Model file for the job. Use its own axes, mm. Round coordinates to 2 decimals unless told otherwise and drop trailing zeros. Loops run counter-clockwise (first coordinate to the right, second up) from the corner with the lowest first, then second, coordinate; pieces in that order, holes last. Notation, with made-up numbers: (-17, 41) - (42, 41) arc R21 ccw to (42, 52) - close; hole circle Ø2 at (23, 59.5). An arc over 180 degrees is marked (long way). Use one line per item in the form item = value.
from build123d import *

# Parameters (mm, degrees)
F1_DEPTH      = 19.05
F2_R          = 3.175
F3_DEPTH      = 19.05
F4_R          = 3.175
F4_R_2        = 1.175
F5_DEPTH      = 304.8
F5_DEPTH_BACK = 19.05


with BuildPart() as f1:
    # F0 (on Top) → F1 (new body)
    with BuildSketch(Plane.XY):
        Polygon((134.8747963854, 77.87), (0, 155.74), (-134.8747963854, 77.87), (-134.8747963854, -77.87), (0, -155.74), (134.8747963854, -77.87), align=None)
    extrude(amount=F1_DEPTH)

    # F2 (on face) → F3 (cut)
    with BuildSketch(Plane.XY.offset(19.05)):
        with BuildLine():
            ThreePointArc((25.4095597529, 94.8297679959), (21.5209947863, 92.5847039657), (23.7660588165, 88.696138999))
            Line((23.7660588165, 88.696138999), (24.5878092847, 91.7629534975))
            Line((24.5878092847, 91.7629534975), (25.4095597529, 94.8297679959))
        make_face()
        with BuildLine():
            ThreePointArc((35.5273806378, 120.7407282861), (30.4195631007, 123.2596251416), (31.5306301696, 117.6739137877))
            ThreePointArc((31.5306301696, 117.6739137877), (34.2851981749, 118.2218314307), (35.5273806378, 120.7407282861))
        make_face()
        with BuildLine():
            Line((24.5878092847, 91.7629534975), (23.7660588165, 88.696138999))
            ThreePointArc((23.7660588165, 88.696138999), (26.5206268218, 89.244056642), (27.7628092847, 91.7629534975))
            ThreePointArc((27.7628092847, 91.7629534975), (27.1067061402, 93.6957710346), (25.4095597529, 94.8297679959))
            Line((25.4095597529, 94.8297679959), (24.5878092847, 91.7629534975))
        make_face()
        with Locations((-24.5878092847, 91.7629534975)):
            Circle(F2_R)
        with Locations((-32.3523806378, 120.7407282861)):
            Circle(F2_R)
        with Locations((-67.1751442127, 67.1751442127)):
            Circle(F2_R)
        with Locations((-88.3883476483, 88.3883476483)):
            Circle(F2_R)
        with Locations((-91.7629534975, 24.5878092847)):
            Circle(F2_R)
        with Locations((-120.7407282861, 32.3523806378)):
            Circle(F2_R)
        with Locations((-91.7629534975, -24.5878092847)):
            Circle(F2_R)
        with Locations((-120.7407282861, -32.3523806378)):
            Circle(F2_R)
        with Locations((-67.1751442127, -67.1751442127)):
            Circle(F2_R)
        with Locations((-88.3883476483, -88.3883476483)):
            Circle(F2_R)
        with Locations((-24.5878092847, -91.7629534975)):
            Circle(F2_R)
        with Locations((-32.3523806378, -120.7407282861)):
            Circle(F2_R)
        with Locations((24.5878092847, -91.7629534975)):
            Circle(F2_R)
        with Locations((32.3523806378, -120.7407282861)):
            Circle(F2_R)
        with Locations((67.1751442127, -67.1751442127)):
            Circle(F2_R)
        with Locations((88.3883476483, -88.3883476483)):
            Circle(F2_R)
        with Locations((91.7629534975, -24.5878092847)):
            Circle(F2_R)
        with Locations((120.7407282861, -32.3523806378)):
            Circle(F2_R)
        with Locations((91.7629534975, 24.5878092847)):
            Circle(F2_R)
        with Locations((120.7407282861, 32.3523806378)):
            Circle(F2_R)
        with Locations((67.1751442127, 67.1751442127)):
            Circle(F2_R)
        with Locations((88.3883476483, 88.3883476483)):
            Circle(F2_R)
    extrude(amount=-F3_DEPTH, mode=Mode.SUBTRACT)

    # F4 (on face) → F5 (join, two sides)
    with BuildSketch(Plane.XY.offset(19.05)) as f5_sk:
        with Locations((-88.3883476483, 88.3883476483)):
            Circle(F4_R)
        with Locations((-88.3883476483, 88.3883476483)):
            Circle(F4_R_2, mode=Mode.SUBTRACT)
        with Locations((-67.1751442127, 67.1751442127)):
            Circle(F4_R)
        with Locations((-67.1751442127, 67.1751442127)):
            Circle(F4_R_2, mode=Mode.SUBTRACT)
        with Locations((-120.7407282861, 32.3523806378)):
            Circle(F4_R)
        with Locations((-120.7407282861, 32.3523806378)):
            Circle(F4_R_2, mode=Mode.SUBTRACT)
        with Locations((-91.7629534975, 24.5878092847)):
            Circle(F4_R)
        with Locations((-91.7629534975, 24.5878092847)):
            Circle(F4_R_2, mode=Mode.SUBTRACT)
        with Locations((-120.7407282861, -32.3523806378)):
            Circle(F4_R)
        with Locations((-120.7407282861, -32.3523806378)):
            Circle(F4_R_2, mode=Mode.SUBTRACT)
        with Locations((-91.7629534975, -24.5878092847)):
            Circle(F4_R)
        with Locations((-91.7629534975, -24.5878092847)):
            Circle(F4_R_2, mode=Mode.SUBTRACT)
        with Locations((-88.3883476483, -88.3883476483)):
            Circle(F4_R)
        with Locations((-88.3883476483, -88.3883476483)):
            Circle(F4_R_2, mode=Mode.SUBTRACT)
        with Locations((-67.1751442127, -67.1751442127)):
            Circle(F4_R)
        with Locations((-67.1751442127, -67.1751442127)):
            Circle(F4_R_2, mode=Mode.SUBTRACT)
        with Locations((-32.3523806378, -120.7407282861)):
            Circle(F4_R)
        with Locations((-32.3523806378, -120.7407282861)):
            Circle(F4_R_2, mode=Mode.SUBTRACT)
        with Locations((-24.5878092847, -91.7629534975)):
            Circle(F4_R)
        with Locations((-24.5878092847, -91.7629534975)):
            Circle(F4_R_2, mode=Mode.SUBTRACT)
        with Locations((32.3523806378, -120.7407282861)):
            Circle(F4_R)
        with Locations((32.3523806378, -120.7407282861)):
            Circle(F4_R_2, mode=Mode.SUBTRACT)
        with Locations((24.5878092847, -91.7629534975)):
            Circle(F4_R)
        with Locations((24.5878092847, -91.7629534975)):
            Circle(F4_R_2, mode=Mode.SUBTRACT)
        with Locations((88.3883476483, -88.3883476483)):
            Circle(F4_R)
        with Locations((88.3883476483, -88.3883476483)):
            Circle(F4_R_2, mode=Mode.SUBTRACT)
        with Locations((67.1751442127, -67.1751442127)):
            Circle(F4_R)
        with Locations((67.1751442127, -67.1751442127)):
            Circle(F4_R_2, mode=Mode.SUBTRACT)
        with Locations((120.7407282861, -32.3523806378)):
            Circle(F4_R)
        with Locations((120.7407282861, -32.3523806378)):
            Circle(F4_R_2, mode=Mode.SUBTRACT)
        with Locations((91.7629534975, -24.5878092847)):
            Circle(F4_R)
        with Locations((91.7629534975, -24.5878092847)):
            Circle(F4_R_2, mode=Mode.SUBTRACT)
        with Locations((120.7407282861, 32.3523806378)):
            Circle(F4_R)
        with Locations((120.7407282861, 32.3523806378)):
            Circle(F4_R_2, mode=Mode.SUBTRACT)
        with Locations((91.7629534975, 24.5878092847)):
            Circle(F4_R)
        with Locations((91.7629534975, 24.5878092847)):
            Circle(F4_R_2, mode=Mode.SUBTRACT)
        with Locations((88.3883476483, 88.3883476483)):
            Circle(F4_R)
        with Locations((88.3883476483, 88.3883476483)):
            Circle(F4_R_2, mode=Mode.SUBTRACT)
        with Locations((67.1751442127, 67.1751442127)):
            Circle(F4_R)
        with Locations((67.1751442127, 67.1751442127)):
            Circle(F4_R_2, mode=Mode.SUBTRACT)
        with Locations((32.3523806378, 120.7407282861)):
            Circle(F4_R)
        with Locations((32.3523806378, 120.7407282861)):
            Circle(F4_R_2, mode=Mode.SUBTRACT)
        with Locations((24.5878092847, 91.7629534975)):
            Circle(F4_R)
        with Locations((24.5878092847, 91.7629534975)):
            Circle(F4_R_2, mode=Mode.SUBTRACT)
        with Locations((-32.3523806378, 120.7407282861)):
            Circle(F4_R)
        with Locations((-32.3523806378, 120.7407282861)):
            Circle(F4_R_2, mode=Mode.SUBTRACT)
        with Locations((-24.5878092847, 91.7629534975)):
            Circle(F4_R)
        with Locations((-24.5878092847, 91.7629534975)):
            Circle(F4_R_2, mode=Mode.SUBTRACT)
    extrude(amount=F5_DEPTH)
    extrude(f5_sk.sketch, amount=-F5_DEPTH_BACK)


solid = f1.part
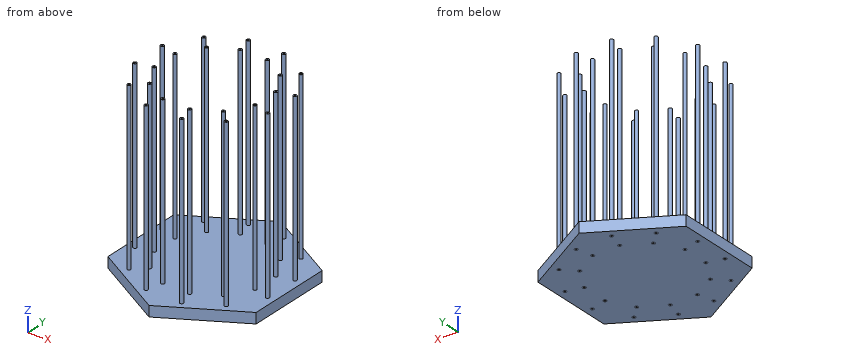
1. Cut at A-A, the plane z = 146. Give the number of separate pieces and of enclosed holes in the cut face, plus the area to 3 significant figures.
Geometry check:
separate_pieces = 24
enclosed_holes = 24
area = 656 mm^2
2. Cut at B-B, the plane y = -4. Give the cut face in (x, z).
Geometry check:
outline = (-134.87, 0) - (134.87, 0) - (134.87, 19.05) - (-134.87, 19.05) - close
3. Wall check: probe 1 along Y at (x, z) = (-88, 32.5); probe 2 along X at (y, z) = (120, 289.5) (1 decimal); probe 3 along Z at (x, y) = (-69, -20). Give the ranges that are in metal, low to high.
Geometry check:
probe_1 = -91.54 to -89.5, -87.28 to -85.24, 85.24 to 87.28, 89.5 to 91.54
probe_2 = -35.4 to -33.3, -31.4 to -29.3, 29.3 to 31.4, 33.3 to 35.4
probe_3 = 0 to 19.05
4. Flat gauge pins, fed straight in: pin 1 (4 mm diameter, centred on y = -71.5, z = 96, fed in from -X); pin 2 (1.5 mm diameter, centred on x = -87.5, z = 211.5, fed in from -Y); pin 3 (12 mm diameter, centred on y = 119, z = 102.5, fed in from -X). Where does each tip first touch, or does it go through?
Geometry check:
pin_1 = -69.34
pin_2 = -91.56
pin_3 = -35.53
5. Cut at C-C, the plane x = 59. Give the cut face in (y, z), plus the area to 3 significant figures.
Geometry check:
outline = (-121.68, 0) - (121.68, 0) - (121.68, 19.05) - (-121.68, 19.05) - close
area = 4,640 mm^2
